The model under review builds one solid part; all positions refer to its coordinate system, in mm. Round coordinates to 2 decimals unless told otherwise and drop trailing zeros. Loops run counter-clockwise (first coordinate to the right, second up) from the corner with the lowest first, then second, coordinate; pieces in that order, holes last. Notation, with made-up numbers: (39, 67) -> (60, 67) arc R14 ccw to (60, 84) -> close; hole circle Ø10 at (32, 16.5). An arc over 180 degrees is marked (long way). Use a Markdown table: item, result. Add a question column.
1) Consider section C-C on z = 16. Give the boundary of the cut face in (x, y), plus the area to 3 significant figures.
2) Mouldability with a two-part tool opening along X and no side actions: class faces 1 (the flat face through (0, -50, -4)), 2 (the flat face through (-35, 1, 0)), 3 (the flat face through (10, -1, 10)), 4 (the flat face through (-10, -1, 10)) as released by +X, released by -X, zero draft, split by the parting line, or undercut.
3) Consider section B-B on y = -23.5. Give the boundary of the cut face in (x, z).
4) Wall thickness on probe 1 along X at (y, z) = (-29, 0.5); probe 2 along X at (y, z) = (20, 15.5); probe 3 along Z at (x, y) = (-14, 29.5): over which ranges is each line inside the solid? List them lowest first.
5) Consider section A-A on z = 9.5. Give the boundary of the cut face in (x, y), plus the area to 3 significant figures.
6) Consider section D-D on x = -12.5. Give the boundary of the cut face in (y, z).
Solid Edge part; units mm, degrees
sketch "Sketch1" plane through (0, 0, 0) normal (0, -1, 0) x (1, 0, 0)
  line L0 (-35, -20) -> (35, -20)
  line L1 (35, -20) -> (35, 20)
  line L2 (35, 20) -> (-35, 20)
  line L3 (-35, 20) -> (-35, -20)
  dimension "D1" = 35
  dimension "D2" = 35
extrude "Protrusion1" add sketch "Sketch1" along normal mid plane 100
sketch "Sketch2" plane through (0, -50, 0) normal (0, -1, 0) x (1, 0, 0)
  line L0 (0, 0) -> (-20, 20)
  line L1 (-20, 20) -> (20, 20)
  line L2 (20, 20) -> (0, 0)
  dimension "D1" = 20
extrude "Cutout1" cut sketch "Sketch2" against normal through all
Result set:
| question | item | result |
|---|---|---|
| 1 | outline | (-35, -50) -> (-16, -50) -> (-16, 50) -> (-35, 50) -> close; (16, -50) -> (35, -50) -> (35, 50) -> (16, 50) -> close |
| 1 | area | 3,800 mm2 |
| 2 | face 1 | zero draft |
| 2 | face 2 | released by -X |
| 2 | face 3 | undercut |
| 2 | face 4 | undercut |
| 3 | outline | (-35, -20) -> (35, -20) -> (35, 20) -> (20, 20) -> (0, 0) -> (-20, 20) -> (-35, 20) -> close |
| 4 | probe 1 | -35 to -0.5, 0.5 to 35 |
| 4 | probe 2 | -35 to -15.5, 15.5 to 35 |
| 4 | probe 3 | -20 to 14 |
| 5 | outline | (-35, -50) -> (-9.5, -50) -> (-9.5, 50) -> (-35, 50) -> close; (9.5, -50) -> (35, -50) -> (35, 50) -> (9.5, 50) -> close |
| 5 | area | 5,100 mm2 |
| 6 | outline | (-50, -20) -> (50, -20) -> (50, 12.5) -> (-50, 12.5) -> close |
